```python
from build123d import *

# Parameters (mm, degrees)
SKETCH_4_R          = 12.5
CUT_EXTRUDE_1_DEPTH = 5
SKETCH_5_R          = 7.1
CUT_EXTRUDE_2_DEPTH = 92.203487258


with BuildPart() as part:
    # 草图2 → 旋转1 (revolve)
    with BuildSketch(Plane.XY, mode=Mode.PRIVATE) as revolve_1_sk:
        Polygon((0, 0), (-30, 0), (-53.094010768, -40), (-56.094010768, -40), (-28.958548116, 7), (0, 7), align=None)
    revolve(revolve_1_sk.sketch.rotate(Axis((0, 0, 0), (0, 1, 0)), 270), axis=Axis((0, 0, 0), (0, 1, 0)))

    # 草图4 → 切除-拉伸1 (cut)
    with BuildSketch(Plane.XZ):
        with Locations(Location((0, 0, 0), (0, 0, 270))):
            Circle(SKETCH_4_R)
    extrude(amount=-CUT_EXTRUDE_1_DEPTH, mode=Mode.SUBTRACT)

    # 草图5 → 切除-拉伸2 (cut, through all)
    with BuildSketch(Plane.XZ.offset(-5)):
        with Locations(Location((0, 0, 0), (0, 0, 270))):
            Circle(SKETCH_5_R)
    extrude(amount=-CUT_EXTRUDE_2_DEPTH, mode=Mode.SUBTRACT)


solid = part.part
```
Geometry check sheet. Reference: the model listing, model coordinates, mm. A direction names the side the tool comes from. Coordinates: 2 decimals unless noted, no trailing zeros. Loops run counter-clockwise (first coordinate to the right, second up) from the corner with the lowest first, then second, coordinate; pieces in that order, holes last. Notation, with made-up numbers: (72.5, -22.5) -> (125.5, -22.5) arc R34 ccw to (125.5, 14.5) -> close; hole circle Ø11 at (-22.75, 42.25). An arc over 180 degrees is marked (long way). Put each result on its own line as item: value.
1) Cross-section at C-C on y = -28. Record the boundary of the cut face in (x, z), plus the area to 3 significant figures.
Result set:
outline: circle Ø98.33 at (0, 0); hole circle Ø92.33 at (0, 0)
area: 898 mm^2
2) Thickness scan on line 1 (X direction, y = 1.9, z = 0); line 2 (X direction, y = -34, z = -16); line 3 (Y direction, x = -17.5, z = -13). Record the ranges inside material, lowest first.
Result set:
line 1: x = -31.9 to -12.5, 12.5 to 31.9
line 2: x = -50.14 to -46.98, 46.98 to 50.14
line 3: y = 0 to 7
3) Release check for a two-part mould opening along X. For faces 1 (the conical face through (-30.018, 4.718, 3.941)), 2 (the flat face through (6, 7, -6)), 3 (the flat face through (13, 0, 0)) record: released by +X, released by -X, zero draft, split by the parting line, or undercut.
Result set:
face 1: split by the parting line
face 2: zero draft
face 3: undercut
4) Cross-section at B-B on z = 0. Record the boundary of the cut face in (x, y).
Result set:
outline: (-56.09, -40) -> (-53.09, -40) -> (-30, 0) -> (-12.5, 0) -> (-12.5, 5) -> (-7.1, 5) -> (-7.1, 7) -> (-28.96, 7) -> close; (7.1, 5) -> (12.5, 5) -> (12.5, 0) -> (30, 0) -> (53.09, -40) -> (56.09, -40) -> (28.96, 7) -> (7.1, 7) -> close
5) Cross-section at A-A on x = 0. Record the boundary of the cut face in (y, z), plus the area to 3 significant figures.
Result set:
outline: (-40, -56.09) -> (7, -28.96) -> (7, -7.1) -> (5, -7.1) -> (5, -12.5) -> (0, -12.5) -> (0, -30) -> (-40, -53.09) -> close; (-40, 53.09) -> (0, 30) -> (0, 12.5) -> (5, 12.5) -> (5, 7.1) -> (7, 7.1) -> (7, 28.96) -> (-40, 56.09) -> close
area: 520 mm^2
6) Cross-section at D-D on y = 1.5. Record the boundary of the cut face in (x, z), plus the area to 3 significant figures.
Result set:
outline: circle Ø64.27 at (0, 0); hole circle Ø25 at (0, 0)
area: 2,750 mm^2
7) Gauge pin test, flat ends, axial feed: pin 1 Ø1.5 at (y, z) = (-17, -12.5) entering from +X; pin 2 Ø1.5 at (y, z) = (-1, -6.5) entering from +X; pin 3 Ø3 at (x, y) = (14, 0.5) entering from +Z; pin 4 Ø22.5 at (x, z) = (0, 0) entering from +Y. Record the tip position at first contact, or that the pin passes through.
Result set:
pin 1: stops at x = 41.45
pin 2: stops at x = 33.41
pin 3: stops at z = 30.73
pin 4: stops at y = 7
8) Tool access check on faces 4 (the flat face through (-5.4, 5, -5.4)), 5 (the flat face through (41, -40, -34)). Record the directions out of +Z, -Z, +X, -X, +Y, -Y that give a thin tool (end or side, any length) a straight path to the whole face; none if there is none.
Result set:
face 4: -Y
face 5: +Z, -Z, +X, -X, -Y
